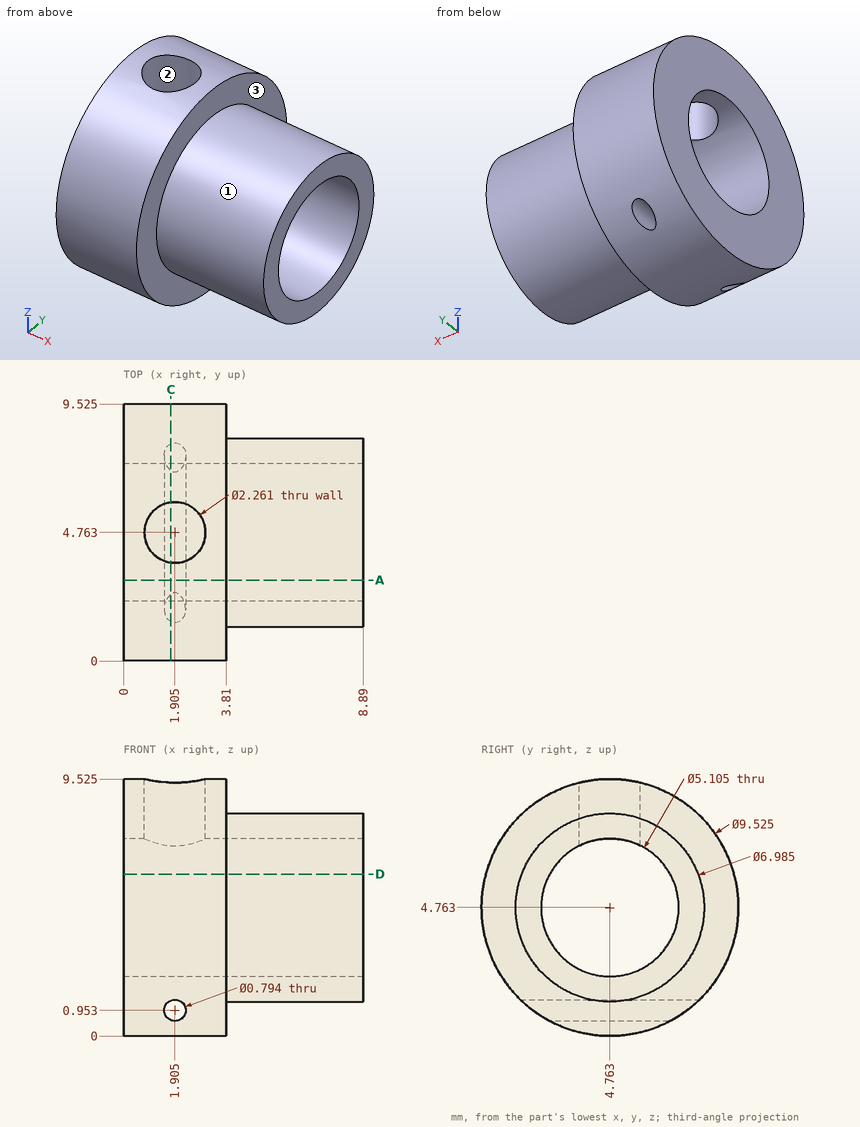
Verification items for this drawing (mm, ordinates from the low corner). Round coordinates to 2 decimals unless told otherwise and drop trailing zeros. Order: outer loops, then holes, each group sorted by start corner. A loop starts at its lowest first (then second) coordinate and runs counter-clockwise, first axis right, second up. Notation, with made-up numbers: M 83,-33.75 L 106,-33.75 A7 ccw 106,-20.75 Z; hole C -0.75,13.5 d9. An arc over 180 degrees is marked long. Answer in a Markdown table with one row per item. Add a question column.
Item 1: Depth check by flat-ended pin: pin 1 Ø5 at (y, z) = (4, 7) entering from -X; pin 2 Ø1 at (x, z) = (4.5, 5) entering from +Y (1 decimal); pin 3 Ø4 at (y, z) = (4.76, 4.76) entering from +X. Enter the tip coordinate at first touch or a pass-through.
Item 2: Sectioned sample at C-C, the plane x = 1.75. Enter the section's corners in (y, z) (1 decimal).
Item 3: Draft check along X on the marked faces 1, 2 and 3. Enter one of: released by +X, released by -X, zero draft, split by the parting line, or undercut.
Item 4: Sectioned sample at D-D, the plane z = 6. Enter the section's corners in (x, y) (1 decimal).
Item 5: Sectioned sample at A-A, the plane y = 3. State how many separate pieces and enclosed holes the cut face has.
Item 6: Material ranges on L1, parallel to X at y = 8, z = 1.75; L2, parallel to Y at x = 7.5, z = 5 (1 decimal); L3, parallel to Y at x = 0.5, z = 5 (1 decimal), recorded low to high. Write a range as [from, to].
Filled in:
| question | item | result |
|---|---|---|
| 1 | pin 1 | stops at x = 0 |
| 1 | pin 2 | stops at y = 8.3 |
| 1 | pin 3 | passes through |
| 2 | outline | M 1.5,1.3 L 8.1,1.3 A4.8 ccw 5.9,9.4 L 5.9,7.1 A2.6 cw long 3.6,7.1 L 3.6,9.4 A4.8 ccw Z; M 2.5,0.6 A4.8 ccw 7.1,0.6 Z |
| 3 | face 1 | zero draft |
| 3 | face 2 | undercut |
| 3 | face 3 | released by +X |
| 4 | outline | M 0,0.2 L 3.8,0.2 L 3.8,1.5 L 8.9,1.5 L 8.9,2.5 L 0,2.5 Z; M 0,7 L 8.9,7 L 8.9,8 L 3.8,8 L 3.8,9.4 L 0,9.4 Z |
| 5 | separate pieces | 2 |
| 5 | enclosed holes | 1 |
| 6 | L1 | x = [0, 3.81] |
| 6 | L2 | y = [1.3, 2.2], [7.3, 8.2] |
| 6 | L3 | y = [0, 2.2], [7.3, 9.5] |
